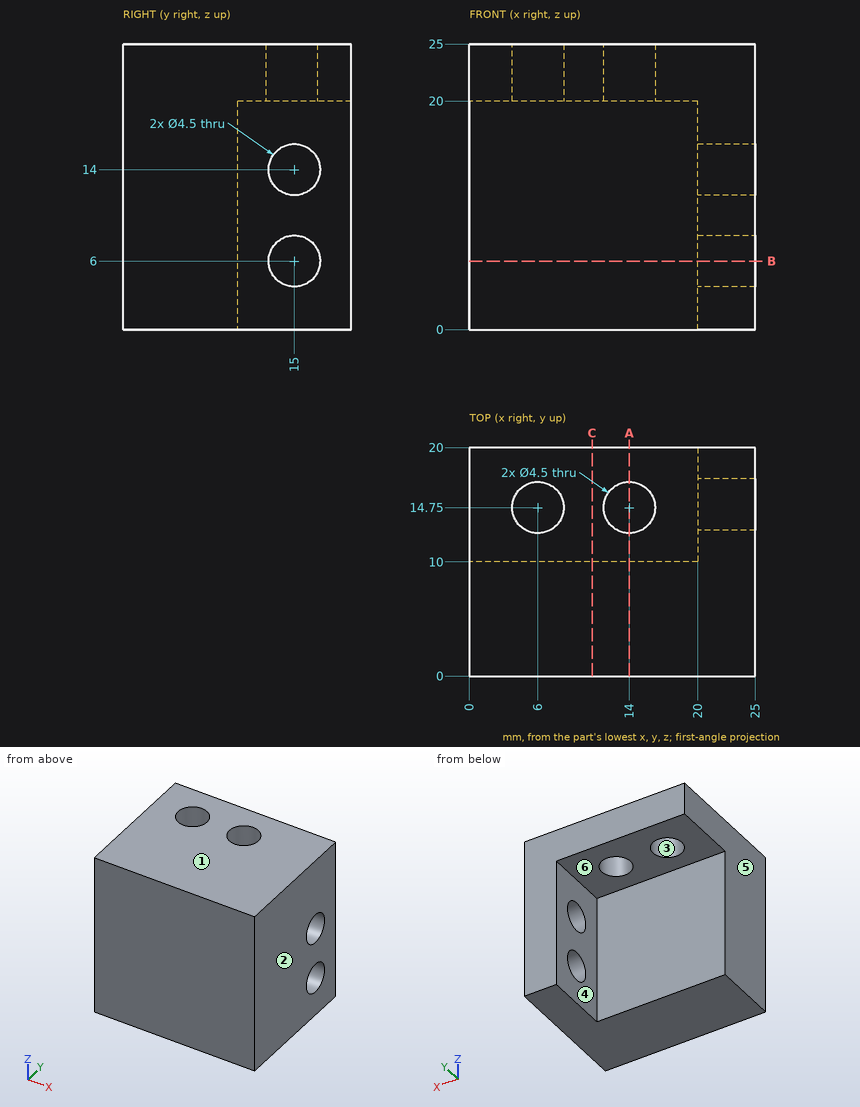
Source: three-view drawing plus pictorial views. Frame: mm from the lowest corner of the part. A direction names the side the tool comes from. Round coordinates to 2 decimals unless told otherwise and drop trailing zeros. Loops run counter-clockwise (first coordinate to the right, second up) from the corner with the lowest first, then second, coordinate; pieces in that order, holes last. Notation, with made-up numbers: M 13,64.5 L 29,64.5 A13 cw 29,82.5 Z; hole C 77,-34.75 d8. An arc over 180 degrees is marked long. Put each result on its own line as item: value. Start each with the question number.
(1) Section query A-A (x = 14). Return loops of the section in (y, z).
(2) Section query C-C (x = 10.75). Return loops of the section in (y, z).
(3) Section query B-B (z = 6). Return loops of the section in (x, y), then the cut area to 4 significant figures.
(4) Contact query for flat-ended pins moving along their axis: pin 1 Ø4 at (y, z) = (15, 6) entering from +X; pin 2 Ø4 at (y, z) = (8, 15) entering from -X; pin 3 Ø3 at (y, z) = (12.5, 11) entering from -X; pin 4 Ø5 at (x, y) = (12, 16.5) entering from -Z. Output: stop coordinate, or through.
(5) Draft query along X for the marked faces 1, 2, 3 and 4. Return one class per face: +X half, -X half, draft (parallel to the pull), parting line (faces both ways), or undercut.
(6) Set-up query: the marked faces 5 and 6. Return all of +Z, -Z, +X, -X, +Y, -Y with unobstructed straight access to the full face (end or side cutting, diameter ignored); none if empty.
(7) Material intervals for line 1 along Y through (x, z) = (14, 23.8); line 2 along Z through (x, y) = (23.75, 15.5); line 3 along Z through (x, y) = (10.25, 14.75), sorted ascending. Write a range as [from, to].
Findings below:
1. outline: M 0,0 L 10,0 L 10,20 L 12.5,20 L 12.5,25 L 0,25 Z; M 17,20 L 20,20 L 20,25 L 17,25 Z
2. outline: M 0,0 L 10,0 L 10,20 L 20,20 L 20,25 L 0,25 Z
3. outline: M 0,0 L 25,0 L 25,12.75 L 20,12.75 L 20,10 L 0,10 Z; M 20,17.25 L 25,17.25 L 25,20 L 20,20 Z
3. area: 277.5 mm2
4. pin 1: passes through
4. pin 2: stops at x = 0
4. pin 3: stops at x = 20
4. pin 4: stops at z = 20
5. face 1: draft
5. face 2: +X half
5. face 3: undercut
5. face 4: -X half
6. face 5: +Z, -Z, -X, +Y, -Y
6. face 6: -Z, -X, +Y
7. line 1: y = [0, 12.5], [17, 20]
7. line 2: z = [0, 3.81], [8.19, 11.81], [16.19, 25]
7. line 3: z = [20, 25]
